from build123d import *

# Parameters (mm, degrees)
SKIZZE1_R                       = 35
AUFSATZ_LINEAR_AUSTRAGEN2_DEPTH = 140
AU_ENGEWINDE_R                  = 3
AUFSATZ_LINEAR_AUSTRAGEN4_DEPTH = 10
KERNLOCH_F_R_M4X0_71_D          = 3.3
KERNLOCH_F_R_M4X0_71_DEPTH      = 15
KERNLOCH_F_R_M4X0_71_TIP        = 0.991420021


with BuildPart() as part:
    # Skizze1 → Aufsatz-Linear austragen2 (new body)
    with BuildSketch(Plane(origin=(0, 0, 0), x_dir=(1, 0, 0), z_dir=(0, 1, 0))):
        with Locations(Location((0, 0, 0), (0, 0, 270))):
            Circle(SKIZZE1_R)
    extrude(amount=AUFSATZ_LINEAR_AUSTRAGEN2_DEPTH)

    # Außengewinde → Aufsatz-Linear austragen4 (add)
    with BuildSketch(Plane.XZ):
        with Locations(Location((0, 0, 0), (0, 0, 90))):
            Circle(AU_ENGEWINDE_R)
    extrude(amount=AUFSATZ_LINEAR_AUSTRAGEN4_DEPTH)

    # Kernloch für M4x0.71
    with Locations(Plane(origin=(0, 140, 0), x_dir=(1, 0, 0), z_dir=(0, 1, 0))):
        with Locations((0, 0)):
            Hole(KERNLOCH_F_R_M4X0_71_D / 2, depth=KERNLOCH_F_R_M4X0_71_DEPTH)
            with Locations((0, 0, -(KERNLOCH_F_R_M4X0_71_DEPTH + KERNLOCH_F_R_M4X0_71_TIP / 2))):  # 118° drill point
                Cone(0, KERNLOCH_F_R_M4X0_71_D / 2, KERNLOCH_F_R_M4X0_71_TIP, mode=Mode.SUBTRACT)


solid = part.part
Geometry check sheet. Reference: the model listing, model coordinates, mm. A direction names the side the tool comes from. Give positions to 0.01 mm unless a question says otherwise; leave off trailing zeros. Order: outer loops, then holes, each group sorted by start corner. A loop starts at its lowest first (then second) coordinate and runs counter-clockwise, first axis right, second up.
1. Access from +Z, -Z, +X, -X, +Y, -Y to the whole of each face (thin tool, end or side, straight path). Record for faces 1 (the face through (1.216, 132.395, -1.115)), 2 (the face through (0, -10, 0)), 3 (the face through (-0.9, -4.93, 2.86)).
Completed:
face 1: +Y
face 2: +Z, -Z, +X, -X, -Y
face 3: -Y
2. Sectioned sample at A-A (x = -12). Record the boundary of the cut face in (y, z).
Completed:
outline: (0, -32.88) - (140, -32.88) - (140, 32.88) - (0, 32.88) - close
3. Scan lines: line 1 (Y direction, x = -30, z = -15); line 2 (X direction, y = 63.5, z = -0.5); line 3 (Z direction, x = 1.5, y = 9.5). Record each from-to range of solid material in increasing order.
Completed:
line 1: y = 0 to 140
line 2: x = -35 to 35
line 3: z = -34.97 to 34.97
4. Sectioned sample at C-C (z = -18.5). Record the boundary of the cut face in (x, y).
Completed:
outline: (-29.71, 0) - (29.71, 0) - (29.71, 140) - (-29.71, 140) - close
5. Depth check by flat-ended pin: pin 1 (1 mm diameter, centred on x = 3.5, z = -6.5, fed in from -Y); pin 2 (2 mm diameter, centred on x = 21.5, y = 105.5, fed in from +Z); pin 3 (4 mm diameter, centred on y = 33, z = -9, fed in from +X). Enter the tip coordinate at first touch or a pass-through.
Completed:
pin 1: stops at y = 0
pin 2: stops at z = 28.37
pin 3: stops at x = 34.29
6. Sectioned sample at B-B (y = 37). Record the boundary of the cut face in (x, z), then the cut area to 3 significant figures.
Completed:
outline: circle Ø70 at (0, 0)
area: 3,850 mm2
7. Draft check along Z on faces 4 (the face through (-21, 69, -28)), 5 (the face through (-7, 140, 0)), 6 (the face through (-0.1, 124.2, 0.3)). Enter one of: pulls with the +Z half, pulls with the -Z half, needs draft (parallel to the pull), parting line crosses it, or undercut.
Completed:
face 4: parting line crosses it
face 5: needs draft
face 6: undercut
